Source: CAD feature listing. Evaluate the final solid. Frame: model axes, mm. A direction names the side the tool comes from. Coordinates: 2 decimals unless noted, no trailing zeros. Loops run counter-clockwise (first coordinate to the right, second up) from the corner with the lowest first, then second, coordinate; pieces in that order, holes last.
Item 1: Section query C-C, the plane z = 27. Return the cut outline in (x, y).
Item 2: Section query A-A, the plane x = 0. Return the cut outline in (y, z).
Item 3: Pull-direction query (X, two-part tool) for faces 4 (the flat face through (19.05, -1, 73)), 5 (the flat face through (-5, 26, 69.85)), 6 (the flat face through (5, 0, 6.35)); classes: +X half, -X half, draft (parallel to the pull), parting line (faces both ways), or undercut.
Item 4: Reachability of faces 1 (the cylindrical face through (-2.75, -12.4, 41.76)), 2 (the flat face through (9.652, 43, 73)), 3 (the cylindrical face through (-15.12, -11.59, 34.44)) from +Z, -Z, +X, -X, +Y, -Y: full face, straight path, thin tool, end or side. Return the list, or none.
Item 5: Line query: probe 1 along X at (y, z) = (0, 1.5); probe 2 along Y at (x, z) = (0, 62.5); probe 3 along Z at (x, y) = (14, 13.5). Output: solid intervals per line, ascending.
Item 6: Section query B-B, the plane y = 31.5. Return the cut outline in (x, z), then the cut area to 3 significant figures.
Item 7: Pin query (flat end, axial travel): pin 1 Ø5 at (x, z) = (-5, 49.5) entering from -Y; pin 2 Ø10 at (x, z) = (-0.5, 67) entering from +Y; pin 3 Ø1.9 at (x, z) = (-12.5, 74.5) entering from +Y. Return the tip coordinate at first contact, or that it passes through.
Item 8: Section query D-D, the plane y = -31. Return the cut outline in (x, z), then the cut area to 3 significant figures.
```python
from build123d import *

# Parameters (mm, degrees)
F0_R     = 19.05
F1_DEPTH = 69.85
F2_R     = 12.7
F3_DEPTH = 63.5
F4_R     = 4.7625
F5_DEPTH = 69.851
F7_DEPTH = 6.35
F8_R     = 12.7
F9_DEPTH = 6.35


with BuildPart() as f1:
    # F0 (on Top) → F1 (new body)
    with BuildSketch(Plane.XY):
        Circle(F0_R)
    extrude(amount=F1_DEPTH)

    # F2 (on face) → F3 (cut)
    with BuildSketch(Plane.XY.offset(69.85)):
        Circle(F2_R)
    extrude(amount=-F3_DEPTH, mode=Mode.SUBTRACT)

    # F4 (on face) → F5 (cut, through all)
    with BuildSketch(Plane(origin=(0, 0, 0), x_dir=(1, 0, 0), z_dir=(0, 0, -1))):
        Circle(F4_R)
    extrude(amount=-F5_DEPTH, mode=Mode.SUBTRACT)

    # F6 (on face) → F7 (join)
    with BuildSketch(Plane.XY.offset(69.85)):
        with BuildLine():
            ThreePointArc((-17.526, 50.7907223972), (-18.6036307345, 50.3443531317), (-19.05, 49.2667223972))
            Line((-19.05, 49.2667223972), (-19.05, -49.276))
            ThreePointArc((-19.05, -49.276), (-18.6036307345, -50.3536307345), (-17.526, -50.8))
            Line((-17.526, -50.8), (-9.652, -50.8))
            Line((-9.652, -50.8), (-9.652, -35.052))
            ThreePointArc((-9.652, -35.052), (0, -25.4), (9.652, -35.052))
            Line((9.652, -35.052), (9.652, -50.8))
            Line((9.652, -50.8), (17.526, -50.8))
            ThreePointArc((17.526, -50.8), (18.6036307345, -50.3536307345), (19.05, -49.276))
            Line((19.05, -49.276), (19.05, 49.276))
            ThreePointArc((19.05, 49.276), (18.6036307345, 50.3536307345), (17.526, 50.8))
            Line((17.526, 50.8), (9.652, 50.8))
            Line((9.652, 50.8), (9.652, 35.052))
            ThreePointArc((9.652, 35.052), (0, 25.4), (-9.652, 35.052))
            Line((-9.652, 35.052), (-9.652, 50.7907223972))
            Line((-9.652, 50.7907223972), (-17.526, 50.7907223972))
        make_face()
    extrude(amount=F7_DEPTH)

    # F8 (on face) → F9 (cut)
    with BuildSketch(Plane.XY.offset(76.2)):
        Circle(F8_R)
    extrude(amount=-F9_DEPTH, mode=Mode.SUBTRACT)


solid = f1.part
```
Verdict:
1. outline: circle Ø38.1 at (0, 0); hole circle Ø25.4 at (0, 0)
2. outline: (-25.4, 69.85) - (-19.05, 69.85) - (-19.05, 0) - (-4.76, 0) - (-4.76, 6.35) - (-12.7, 6.35) - (-12.7, 76.2) - (-25.4, 76.2) - close; (4.76, 0) - (19.05, 0) - (19.05, 69.85) - (25.4, 69.85) - (25.4, 76.2) - (12.7, 76.2) - (12.7, 6.35) - (4.76, 6.35) - close
3. face 4: +X half
3. face 5: draft
3. face 6: undercut
4. face 1: +Z
4. face 2: +Z, -Z, +Y
4. face 3: -Z
5. probe 1: x = -19.05 to -4.76, 4.76 to 19.05
5. probe 2: y = -19.05 to -12.7, 12.7 to 19.05
5. probe 3: z = 69.85 to 76.2
6. outline: (-19.05, 69.85) - (-8.97, 69.85) - (-8.97, 76.2) - (-19.05, 76.2) - close; (8.97, 69.85) - (19.05, 69.85) - (19.05, 76.2) - (8.97, 76.2) - close
6. area: 128 mm2
7. pin 1: stops at y = -18.89
7. pin 2: stops at y = 26.57
7. pin 3: stops at y = 50.79
8. outline: (-19.05, 69.85) - (-8.76, 69.85) - (-8.76, 76.2) - (-19.05, 76.2) - close; (8.76, 69.85) - (19.05, 69.85) - (19.05, 76.2) - (8.76, 76.2) - close
8. area: 131 mm2
